Check sheet for the drawn part. Datum: minimum x, y, z corner. Units: mm. A direction names the side the tool comes from. Give positions to 0.01 mm unless a question says otherwise; leave off trailing zeros. Order: outer loops, then holes, each group sorted by start corner. A loop starts at its lowest first (then second) coordinate and runs counter-clockwise, first axis right, second up. Notation, with made-up numbers: (-19, 53.5) -> (-8, 53.5) arc R21 ccw to (-8, 74.5) -> close; hole circle Ø11 at (-32.75, 51). An arc over 180 degrees is marked (long way). Answer in a Markdown table with one row per item. Add a question column.
(1) Set-up check for the marked faces 4, 5 and 6: record each of +Z, -Z, +X, -X, +Y, -Y from which the full face is reachable in a straight line by a thin tool's end or side.
(2) Cross-section at A-A (x = 16.75). Record the cut outline in (y, z), then the cut area to 3 significant figures.
(3) Release check for a two-part mould opening along Z. For the marked faces 1, 2 and 3 record: released by +Z, released by -Z, zero draft, split by the parting line, or undercut.
(4) Thickness scan on L1, parallel to Y at x = 2.3, z = 3.8; L2, parallel to X at y = 15.75, z = 7; L3, parallel to Z at x = 11.5, y = 10.25. Record the ranges inside material, lowest first. Write a range as [from, to].
(5) Cross-section at D-D (z = 6.5). Record the cut outline in (x, y).
(6) Cross-section at C-C (z = 1.5). Record the cut outline in (x, y), then the cut area to 3 significant figures.
(7) Go/stop test with flat-tipped pins: pin 1 (4.5 mm diameter, centred on x = 14.5, z = 8, fed in from -Y); pin 2 (1 mm diameter, centred on x = 15, y = 22, fed in from -Z); pin 3 (3 mm diameter, centred on y = 5, z = 8, fed in from +X). Record where each tip stops, or that it passes through.
(8) Cross-section at B-B (y = 20). Record the cut outline in (x, z), then the cut area to 3 significant figures.
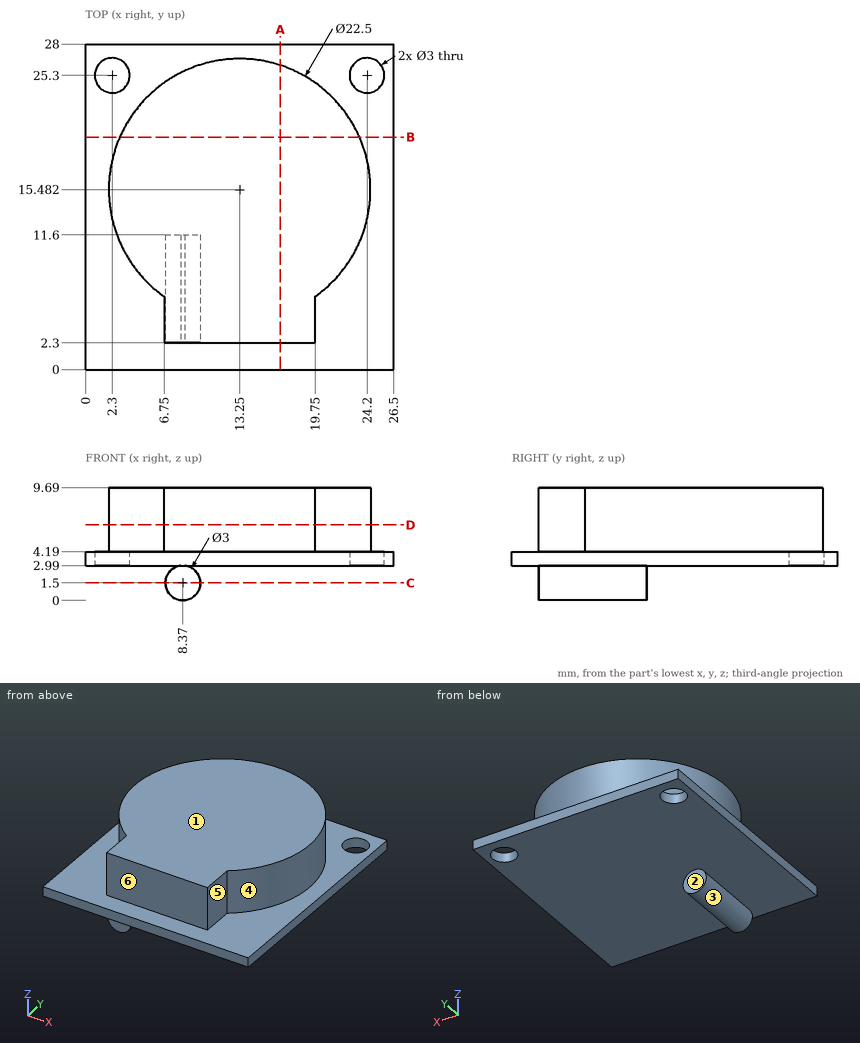
Answer below:
| question | item | result |
|---|---|---|
| 1 | face 4 | +Z |
| 1 | face 5 | +Z, +X, -Y |
| 1 | face 6 | +Z, +X, -X, -Y |
| 2 | outline | (0, 2.99) -> (28, 2.99) -> (28, 4.19) -> (26.17, 4.19) -> (26.17, 9.69) -> (2.3, 9.69) -> (2.3, 4.19) -> (0, 4.19) -> close |
| 2 | area | 165 mm² |
| 3 | face 1 | released by +Z |
| 3 | face 2 | zero draft |
| 3 | face 3 | undercut |
| 4 | L1 | y = [0, 23.8], [26.8, 28] |
| 4 | L2 | x = [2, 24.5] |
| 4 | L3 | z = [2.99, 9.69] |
| 5 | outline | (6.75, 2.3) -> (19.75, 2.3) -> (19.75, 6.3) arc R11.25 ccw (long way) to (6.75, 6.3) -> close |
| 6 | outline | (6.87, 2.3) -> (9.87, 2.3) -> (9.87, 11.6) -> (6.87, 11.6) -> close |
| 6 | area | 27.9 mm² |
| 7 | pin 1 | stops at y = 2.3 |
| 7 | pin 2 | stops at z = 2.99 |
| 7 | pin 3 | stops at x = 20.02 |
| 8 | outline | (0, 2.99) -> (26.5, 2.99) -> (26.5, 4.19) -> (23.55, 4.19) -> (23.55, 9.69) -> (2.95, 9.69) -> (2.95, 4.19) -> (0, 4.19) -> close |
| 8 | area | 145 mm² |
